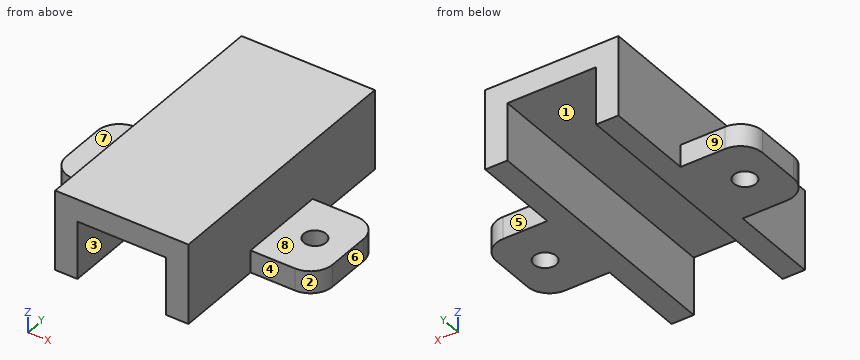
```python
from build123d import *

# Parameters (mm, degrees)
BOSS_EXTRUDE1_DEPTH = 76.2
SKETCH3_R           = 2.5019
BOSS_EXTRUDE2_DEPTH = 6.35
SKETCH4_W           = 19.05
SKETCH4_H           = 25.4
SKETCH4_R           = 3.175
BOSS_EXTRUDE3_DEPTH = 6.35
FILLET1_R           = 6.35
CUT_EXTRUDE1_REACH  = 99.955


with BuildPart() as part:
    # Sketch2 → Boss-Extrude1 (new body)
    with BuildSketch(Plane(origin=(0, 0, 0), x_dir=(1, 0, 0), z_dir=(0, 1, 0))):
        Polygon((0, 22.86), (0, 0), (38.1, 0), (38.1, 22.86), (31.75, 22.86), (31.75, 6.35), (6.35, 6.35), (6.35, 22.86), align=None)
    extrude(amount=BOSS_EXTRUDE1_DEPTH)

    # Sketch3 → Boss-Extrude2 (add)
    with BuildSketch(Plane.XY):
        with BuildLine():
            Line((19.05, 50.8), (-19.05, 50.8))
            ThreePointArc((-19.05, 50.8), (-31.75, 38.1), (-19.05, 25.4))
            Line((-19.05, 25.4), (19.05, 25.4))
            ThreePointArc((19.05, 25.4), (31.75, 38.1), (19.05, 50.8))
        make_face()
        with Locations((-19.05, 38.1)):
            Circle(SKETCH3_R, mode=Mode.SUBTRACT)
    extrude(amount=-BOSS_EXTRUDE2_DEPTH)

    # Sketch4 → Boss-Extrude3 (add)
    # profile 1 of 2: a face of its own
    with BuildSketch(Plane(origin=(0, 0, -22.86), x_dir=(-1, 0, 0), z_dir=(0, 0, -1))):
        with Locations((-47.625, 38.1)):
            Rectangle(SKETCH4_W, SKETCH4_H)
        with Locations((-47.625, 38.1)):
            Circle(SKETCH4_R, mode=Mode.SUBTRACT)
    # profile 2 of 2: a face of its own
    with BuildSketch(Plane(origin=(0, 0, -22.86), x_dir=(-1, 0, 0), z_dir=(0, 0, -1))):
        with Locations((9.525, 38.1)):
            Rectangle(SKETCH4_W, SKETCH4_H)
        with Locations(Location((9.525, 38.1, 0), (0, 0, 180))):
            Circle(SKETCH4_R, mode=Mode.SUBTRACT)
    extrude(amount=-BOSS_EXTRUDE3_DEPTH)

    # Fillet1
    fillet1_edges = [part.edges().sort_by_distance(p)[0] for p in [
        (57.15, 25.4, -19.685),
        (57.15, 50.8, -19.685),
        (-19.05, 50.8, -19.685),
        (-19.05, 25.4, -19.685),
    ]]
    fillet(fillet1_edges, radius=FILLET1_R)

    # Sketch5 → Cut-Extrude1 (cut, up to next)
    with BuildSketch(Plane.XY, mode=Mode.PRIVATE) as cut_extrude1_sk1:
        with BuildLine():
            Line((-19.05, 25.4), (0, 25.4))
            Line((0, 25.4), (0, 50.8))
            Line((0, 50.8), (-19.05, 50.8))
            ThreePointArc((-19.05, 50.8), (-31.75, 38.1), (-19.05, 25.4))
        make_face()
    cut_extrude1_tool1 = extrude(cut_extrude1_sk1.sketch, amount=-CUT_EXTRUDE1_REACH, mode=Mode.PRIVATE) & part.part
    add(cut_extrude1_tool1.solids().sort_by_distance((-14.650694, 38.1, 0))[0], mode=Mode.SUBTRACT)


solid = part.part
```
Could you check a few things on this model? Use its own coordinates, in mm. Face numbers are marked on the shaded views. A direction names the side the tool comes from. Give positions to 0.01 mm unless a question says otherwise; leave off trailing zeros. Loops run counter-clockwise (first coordinate to the right, second up) from the corner with the lowest first, then second, coordinate; pieces in that order, holes last. Notation, with made-up numbers: (5, 25) -> (13, 25) arc R35 ccw to (13, 58) -> close; hole circle Ø1 at (56.25, 0). An arc over 180 degrees is marked (long way). Put each result on its own line as item: value.
(1) Please list where these lines run through material, in increasing order: probe 1 along X at (y, z) = (37, -7.75); probe 2 along X at (y, z) = (35.5, -18); probe 3 along Z at (x, y) = (28, 6). Write a range as [from, to].
Computed:
probe 1: [0, 6.35], [31.75, 38.1]
probe 2: [-19.05, -11.35], [-7.7, 6.35], [31.75, 45.8], [49.45, 57.15]
probe 3: [-6.35, 0]
(2) Imagine slicing it at A-A on z = -8.5. Write out the boundary of the cut face in (x, y), plus the area to 3 significant figures.
Computed:
outline: (0, 0) -> (6.35, 0) -> (6.35, 76.2) -> (0, 76.2) -> close; (31.75, 0) -> (38.1, 0) -> (38.1, 76.2) -> (31.75, 76.2) -> close
area: 968 mm^2
(3) Imagine slicing it at B-B on z = -21. Write out the boundary of the cut face in (x, y) (3 decimals), plus the area to 3 significant figures.
Computed:
outline: (-19.05, 31.75) arc R6.35 ccw to (-12.7, 25.4) -> (0, 25.4) -> (0, 0) -> (6.35, 0) -> (6.35, 76.2) -> (0, 76.2) -> (0, 50.8) -> (-12.7, 50.8) arc R6.35 ccw to (-19.05, 44.45) -> close; (31.75, 0) -> (38.1, 0) -> (38.1, 25.4) -> (50.8, 25.4) arc R6.35 ccw to (57.15, 31.75) -> (57.15, 44.45) arc R6.35 ccw to (50.8, 50.8) -> (38.1, 50.8) -> (38.1, 76.2) -> (31.75, 76.2) -> close; hole circle Ø6.35 at (-9.525, 38.1); hole circle Ø6.35 at (47.625, 38.1)
area: 1,840 mm^2
(4) I'm going to push flat-ended pins straight in: pin 1 Ø9.5 at (x, y) = (48.5, 32) entering from +Z; pin 2 Ø7 at (x, z) = (-7, -20) entering from +Y; pin 3 Ø5 at (y, z) = (66, -11.5) entering from -X. Where does each tip first touch, or does it pass through?
Computed:
pin 1: z = -16.51
pin 2: y = 50.8
pin 3: x = 0
(5) For the marked faces 5, 6, 7, 8 and 9, which set-ups out of +Z, -Z, +X, -X, +Y, -Y let a thin tool reach every point of the face, with its end or its side?
Computed:
face 5: +Z, -Z, +X, +Y
face 6: +Z, -Z, +X, +Y, -Y
face 7: +Z, -X, +Y, -Y
face 8: +Z, +X, +Y, -Y
face 9: +Z, -Z, -X, +Y
(6) Thinking about a two-plate mould opening in X: for the marked faces 1, 2, 3 and 4, which applies, pulls with the +X half, pulls with the -X half, needs draft (parallel to the pull), parting line crosses it, or undercut?
Computed:
face 1: undercut
face 2: pulls with the +X half
face 3: undercut
face 4: needs draft
(7) Imagine slicing it at C-C on y = 38.1. Write out the boundary of the cut face in (x, z).
Computed:
outline: (-19.05, -22.86) -> (-12.7, -22.86) -> (-12.7, -16.51) -> (-19.05, -16.51) -> close; (-6.35, -22.86) -> (6.35, -22.86) -> (6.35, -6.35) -> (31.75, -6.35) -> (31.75, -22.86) -> (44.45, -22.86) -> (44.45, -16.51) -> (38.1, -16.51) -> (38.1, 0) -> (0, 0) -> (0, -16.51) -> (-6.35, -16.51) -> close; (50.8, -22.86) -> (57.15, -22.86) -> (57.15, -16.51) -> (50.8, -16.51) -> close
(8) Imagine slicing it at D-D on y = 65. Write out the boundary of the cut face in (x, z), plus the area to 3 significant figures.
Computed:
outline: (0, -22.86) -> (6.35, -22.86) -> (6.35, -6.35) -> (31.75, -6.35) -> (31.75, -22.86) -> (38.1, -22.86) -> (38.1, 0) -> (0, 0) -> close
area: 452 mm^2
